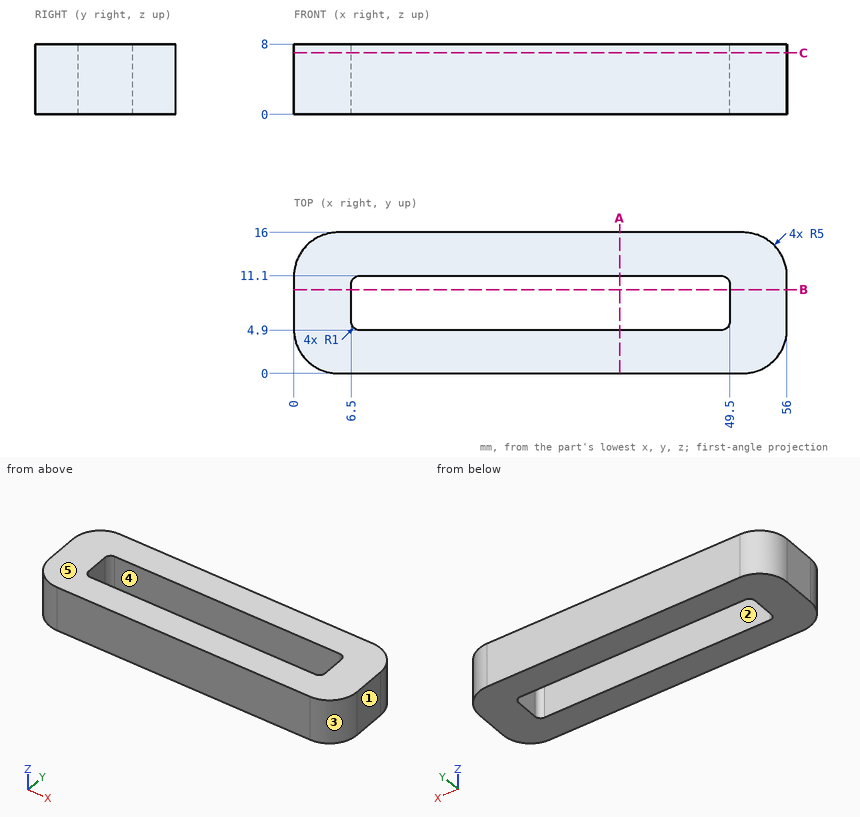
Part print with two shaded views. Sizes in mm from the minimum x, y, z corner. A direction names the side the tool comes from. Coordinates: 2 decimals unless noted, no trailing zeros. Write each loop counter-clockwise with the first axis right and the second up, starting at its lowest first coordinate (ties: lowest second). Pieces come first, ordered by that corner, then holes. Notation, with made-up numbers: (2, 35) -> (27, 35) arc R26 cw to (27, 68) -> close; hole circle Ø6 at (51.25, -15). An arc over 180 degrees is marked (long way). Return JSON: item names as keys, results as strings. Group by question number.
Q1. Which spindle directions (+Z, -Z, +X, -X, +Y, -Y) get a long thin tool onto all of the face, cutting with end or side? Do the marked faces 4 and 5. Say none if no direction does.
Q2. Drill centre lines: line 1 (Y direction, x = 16, z = 7.25); line 2 (X direction, y = 10, z = 1.5); line 3 (X direction, y = 14, z = 7.5). Where is each one in solid material? Low to high.
Q3. Flat gauge pin, fed straight in: pin 1 (3 mm diameter, centred on x = 45.5, y = 11, fed in from -Z). Where does the tip first touch, or does it go through?
Q4. Cut at A-A, the plane x = 37. Give the cut face in (y, z), then the cut area to 3 significant figures.
Q5. Pull direction Y, two halves, no side cores. Call the marked faces 1, 2 and 3: released by +Y, released by -Y, zero draft, split by the parting line, or undercut.
Q6. Cut at C-C, the plane z = 7. Give the cut face in (x, y).
Q7. Cut at B-B, the plane y = 9.5. Give the cut face in (x, z), then the cut area to 3 significant figures.
Returned:
{
 "1": {"face 4": "+Z, -Z", "face 5": "+Z, +X, -X, +Y, -Y"},
 "2": {"line 1": "y = 0 to 4.9, 11.1 to 16", "line 2": "x = 0 to 6.5, 49.5 to 56", "line 3": "x = 1 to 55"},
 "3": {"pin 1": "stops at z = 0"},
 "4": {"outline": "(0, 0) -> (4.9, 0) -> (4.9, 8) -> (0, 8) -> close; (11.1, 0) -> (16, 0) -> (16, 8) -> (11.1, 8) -> close", "area": "78.4 mm2"},
 "5": {"face 1": "zero draft", "face 2": "undercut", "face 3": "released by -Y"},
 "6": {"outline": "(0, 5) arc R5 ccw to (5, 0) -> (51, 0) arc R5 ccw to (56, 5) -> (56, 11) arc R5 ccw to (51, 16) -> (5, 16) arc R5 ccw to (0, 11) -> close; hole (6.5, 5.9) arc R1 ccw to (7.5, 4.9) -> (48.5, 4.9) arc R1 ccw to (49.5, 5.9) -> (49.5, 10.1) arc R1 ccw to (48.5, 11.1) -> (7.5, 11.1) arc R1 ccw to (6.5, 10.1) -> close"},
 "7": {"outline": "(0, 0) -> (6.5, 0) -> (6.5, 8) -> (0, 8) -> close; (49.5, 0) -> (56, 0) -> (56, 8) -> (49.5, 8) -> close", "area": "104 mm2"}
}
